Autodesk Inventor part; units mm, degrees
ref_plane "YZ Plane" through (0, 0, 0) normal (1, 0, 0) x (0, 1, 0)
ref_plane "XZ Plane" through (0, 0, 0) normal (0, 1, 0) x (-1, 0, 0)
ref_plane "XY Plane" through (0, 0, 0) normal (0, 0, 1) x (1, 0, 0)
sketch "Sketch1" plane through (0, 0, 0) normal (0, 1, 0) x (-1, 0, 0)
  circle A0 centre (0, 0) radius 35
  circle A1 centre (0, 0) radius 30
  circle A2 centre (0, -30) radius 2.25
  circle A3 centre (0, 30) radius 2.25
  dimension "d0" = 70
  dimension "d1" = 60
  dimension "d2" = 4.5
  dimension "d3" = 4.5
extrude "Extrusion1" add sketch "Sketch1" along normal mid plane 10 contours A0 | A1 A2 A3
sketch "Sketch2" plane through (0, -5, 0) normal (0, -1, 0) x (1, 0, 0)
  circle A0 centre (0, 0) radius 17.5
  dimension "d6" = 35
extrude "Extrusion2" add sketch "Sketch2" along normal blind 50
properties part number "Adapter Plate"
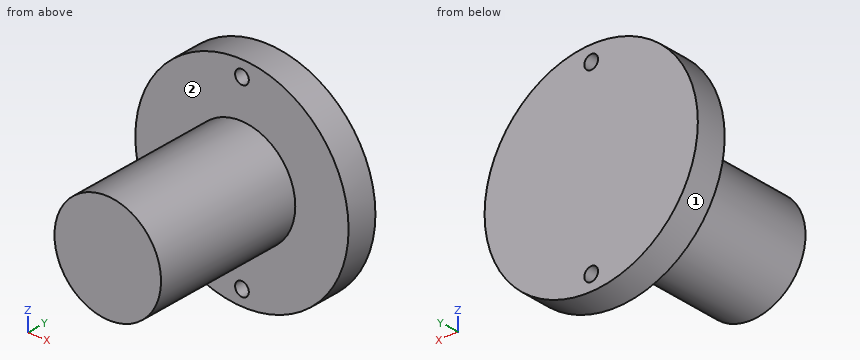
Source: CAD feature listing. Evaluate the final solid. Frame: model axes, mm. Face numbers are marked on the shaded views. A direction names the side the tool comes from. Round coordinates to 2 decimals unless told otherwise and drop trailing zeros. Loops run counter-clockwise (first coordinate to the right, second up) from the corner with the lowest first, then second, coordinate; pieces in that order, holes last. Notation, with made-up numbers: (71, 86.5) -> (128, 86.5) arc R29 ccw to (128, 117.5) -> close; hole circle Ø6 at (-6.5, 70.25). An arc over 180 degrees is marked (long way). Answer as a JSON object with one key per item and string values. Group by question number.
Q1. Section query C-C (z = 0). Output: boundary loops of the cut face in (x, y), plus the area to 3 significant figures.
Q2. Ray query, line 1 (Z direction, x = 0, y = 0.75); line 2 (Y direction, x = 18.5, z = 23); line 3 (X direction, y = 3, z = 30). Return the intervals inside material, ascending. Write a range as from..to.
Q3. Contact query for flat-ended pins moving along their axis: P1, Ø3, axis at y = -17, z = -4, coming from the -X side; P2, Ø8, axis at y = -39, z = 0.5, coming from the +X side; P3, Ø1.5, axis at x = 18.5, z = 26, coming from the -Y side. Output: stop coordinate, or through.
Q4. Access query for the marked faces 1 and 2. Directions: +Z, -Z, +X, -X, +Y, -Y. A direction counts if a zero-diameter tool reaches every point of the face in a straight line with its end or side. Return the directions, or none.
Q5. Section query A-A (x = 0). Output: boundary loops of the cut face in (y, z).
Q6. Section query D-D (x = 28). Output: boundary loops of the cut face in (y, z), plus the area to 3 significant figures.
Q7. Section query B-B (z = 30). Output: boundary loops of the cut face in (x, y).
Completed:
{
 "1": {"outline": "(-35, -5) -> (-17.5, -5) -> (-17.5, -55) -> (17.5, -55) -> (17.5, -5) -> (35, -5) -> (35, 5) -> (-35, 5) -> close", "area": "2,450 mm²"},
 "2": {"line 1": "-35..-32.25, -27.75..27.75, 32.25..35", "line 2": "-5..5", "line 3": "-18.03..-2.25, 2.25..18.03"},
 "3": {"P1": "x = -17.32", "P2": "x = 17.5", "P3": "y = -5"},
 "4": {"face 1": "+Y, -Y", "face 2": "-Y"},
 "5": {"outline": "(-55, -17.5) -> (-5, -17.5) -> (-5, -27.75) -> (5, -27.75) -> (5, 27.75) -> (-5, 27.75) -> (-5, 17.5) -> (-55, 17.5) -> close; (-5, -35) -> (5, -35) -> (5, -32.25) -> (-5, -32.25) -> close; (-5, 32.25) -> (5, 32.25) -> (5, 35) -> (-5, 35) -> close"},
 "6": {"outline": "(-5, -21) -> (5, -21) -> (5, 21) -> (-5, 21) -> close", "area": "420 mm²"},
 "7": {"outline": "(-18.03, -5) -> (-2.25, -5) -> (-2.25, 5) -> (-18.03, 5) -> close; (2.25, -5) -> (18.03, -5) -> (18.03, 5) -> (2.25, 5) -> close"}
}
